Work out the finished part from the listing and answer in its coordinate system (mm). Face numbers are marked on the shaded views. A direction names the side the tool comes from. Give positions to 0.01 mm unless a question says otherwise; leave off trailing zeros. Write each loop counter-clockwise with the first axis right and the second up, starting at its lowest first coordinate (ties: lowest second). Pieces come first, ordered by that corner, then holes. Notation, with made-up numbers: (51.5, -20.5) -> (93.5, -20.5) arc R14 ccw to (93.5, -9.5) -> close; hole circle Ø5 at (63, -2). An arc over 180 degrees is marked (long way). Write item = value, one per line. Start each with the question number.
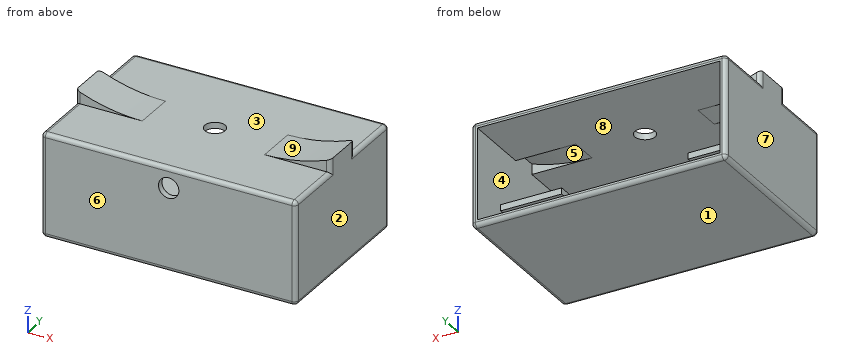
from build123d import *

# Parameters (mm, degrees)
BOSS_EXTRUDE1_DEPTH = 5
BOSS_EXTRUDE2_DEPTH = 20
SHELL1_START        = -18.5
SHELL1_OUTLINE_W    = 59.5
SHELL1_OUTLINE_H    = 22.4
SHELL1_DEPTH        = 38.5
SHELL1_START_2      = -3.5
SHELL1_2_DEPTH      = 7
SKETCH14_R          = 2.5
CUT_EXTRUDE1_DEPTH  = 1.5
SKETCH15_W          = 13.5
SKETCH15_H          = 1.5
SKETCH15_W_2        = 15
BOSS_EXTRUDE3_DEPTH = 10
FILLET21_R          = 1
CUT_EXTRUDE2_START  = -18.5
SKETCH16_R          = 2.5
CUT_EXTRUDE2_DEPTH  = 1.5


# Read off the part's stored shape, not the designer's step: Shell1
with BuildPart() as part:
    # Sketch13 → Boss-Extrude1 (new, symmetric)
    with BuildSketch(Plane(origin=(0, 0, 0), x_dir=(1, 0, 0), z_dir=(0, 1, 0))):
        with BuildLine():
            ThreePointArc((-31.25, 1.770695181), (-23.283883594, 4.184856634), (-15, 5))
            Line((-15, 5), (-31.25, 5))
            Line((-31.25, 5), (-31.25, 1.770695181))
        make_face()
        Polygon((-15, 5), (15, 5), (31.25, 5), (31.25, 30.4), (-31.25, 30.4), (-31.25, 5), align=None)
        with BuildLine():
            Line((31.25, 5), (15, 5))
            ThreePointArc((15, 5), (23.283883594, 4.184856634), (31.25, 1.770695181))
            Line((31.25, 1.770695181), (31.25, 5))
        make_face()
    extrude(amount=BOSS_EXTRUDE1_DEPTH, both=True)

    # Sketch13<12> → Boss-Extrude2 (add, symmetric)
    with BuildSketch(Plane(origin=(0, 0, 0), x_dir=(1, 0, 0), z_dir=(0, 1, 0))):
        Polygon((-15, 5), (15, 5), (31.25, 5), (31.25, 30.4), (-31.25, 30.4), (-31.25, 5), align=None)
    extrude(amount=BOSS_EXTRUDE2_DEPTH, both=True)

    # Shell1 outline → Shell1 (cut)
    with BuildSketch(Plane(origin=(0, 0, 0), x_dir=(1, 0, 0), z_dir=(0, 1, 0)).offset(SHELL1_START)):
        with Locations((0, 17.7)):
            Rectangle(SHELL1_OUTLINE_W, SHELL1_OUTLINE_H)
    extrude(amount=SHELL1_DEPTH, mode=Mode.SUBTRACT)

    # Shell1 2 outline → Shell1 2 (cut)
    with BuildSketch(Plane(origin=(0, 0, 0), x_dir=(1, 0, 0), z_dir=(0, 1, 0)).offset(SHELL1_START_2)):
        with BuildLine():
            Line((-29.75, 6.5), (-29.75, 3.954040816))
            ThreePointArc((-29.75, 3.954040816), (-22.484056523, 5.858838752), (-15, 6.5))
            Line((-15, 6.5), (-29.75, 6.5))
        make_face()
        with BuildLine():
            Line((29.75, 6.5), (15, 6.5))
            ThreePointArc((15, 6.5), (22.484056523, 5.858838752), (29.75, 3.954040816))
            Line((29.75, 3.954040816), (29.75, 6.5))
        make_face()
    extrude(amount=SHELL1_2_DEPTH, mode=Mode.SUBTRACT)

    # Sketch14 → Cut-Extrude1 (cut)
    with BuildSketch(Plane.XY.offset(-5)):
        with Locations(Location((0, 0, 0), (0, 0, 180))):
            Circle(SKETCH14_R)
    extrude(amount=-CUT_EXTRUDE1_DEPTH, mode=Mode.SUBTRACT)

    # Sketch15 → Boss-Extrude3 (add, symmetric)
    with BuildSketch(Plane(origin=(0, 0, 0), x_dir=(1, 0, 0), z_dir=(0, 1, 0))):
        with Locations((-23, 21.15)):
            Rectangle(SKETCH15_W, SKETCH15_H)
        with Locations((22.25, 21.15)):
            Rectangle(SKETCH15_W_2, SKETCH15_H)
    extrude(amount=BOSS_EXTRUDE3_DEPTH, both=True)

    # Fillet21
    fillet21_edges = [part.edges().sort_by_distance(p)[0] for p in [
        (-31.25, 0, -30.4),
        (31.25, 0, -30.4),
        (31.25, -5, -3.385347591),
        (31.25, 5, -3.385347591),
        (31.25, -12.5, -5),
        (-31.25, -20, -17.7),
        (-31.25, -12.5, -5),
        (0, -20, -5),
        (31.25, 12.5, -5),
        (31.25, 20, -17.7),
        (0, 20, -30.4),
        (-31.25, 12.5, -5),
        (-31.25, 20, -17.7),
        (0, 20, -5),
        (31.25, -20, -17.7),
        (0, -20, -30.4),
        (-31.25, 5, -3.385347591),
        (-31.25, -5, -3.385347591),
    ]]
    fillet(fillet21_edges, radius=FILLET21_R)

    # Sketch16 → Cut-Extrude2 (cut)
    with BuildSketch(Plane(origin=(0, 0, 0), x_dir=(1, 0, 0), z_dir=(0, 1, 0)).offset(CUT_EXTRUDE2_START)):
        with Locations(Location((0, 10, 0), (0, 0, 270))):
            Circle(SKETCH16_R)
    extrude(amount=-CUT_EXTRUDE2_DEPTH, mode=Mode.SUBTRACT)


solid = part.part
(1) A cutting plane is placed at C-C, the plane z = -10. Write down the section's boundary in (x, y).
(2) For the marked faces 5, 6, 7, 8 and 9, determine the directions among +Z, -Z, +X, -X, +Y, -Y from which every point of the face is accessible in a straight line to the end or side of a thin tool.
(3) Each of these flat-tipped pins is pushed along its axis until it touches: pin 1 (1.3 mm diameter, centred on x = -25.5, z = -5, fed in from +Y); pin 2 (11 mm diameter, centred on x = -22.5, y = 1.5, fed in from +Z); pin 3 (1 mm diameter, centred on x = 12.5, y = 9, fed in from +Z). Where does it stop, or does it pass through?
(4) A cutting plane is placed at A-A, the plane x = 0. Write down the section's boundary in (y, z), then the cut area to 3 significant figures.
(5) A cutting plane is placed at B-B, the plane y = -8.5. Write down the section's boundary in (x, z), then the cut area to 3 significant figures.
(6) Determine the mould class of the marked faces 1, 2, 3 and 4 for opening direction Z: pulls with the +Z half, pulls with the -Z half, needs draft (parallel to the pull), parting line crosses it, or undercut.
(7) Find the intervals of material crossed by line 1 along Z through (x, y) = (-24.5, -8.5); line 2 along Z through (x, y) = (-12.5, -7); line 3 along X through (y, z) = (14.5, -11), in increasing order.
(8) A cutting plane is placed at D-D, the plane y = 0. Write down the section's boundary in (x, z), then the cut area to 3 significant figures.
Results list:
q1.outline = (-31.25, -19) arc R1 ccw to (-30.25, -20) -> (-2.5, -20) -> (-2.5, -18.5) -> (-29.75, -18.5) -> (-29.75, 20) -> (-30.25, 20) arc R1 ccw to (-31.25, 19) -> close; (2.5, -20) -> (30.25, -20) arc R1 ccw to (31.25, -19) -> (31.25, 19) arc R1 ccw to (30.25, 20) -> (29.75, 20) -> (29.75, -18.5) -> (2.5, -18.5) -> close
q2.face_5 = none
q2.face_6 = +Z, -Z, +X, -X, -Y
q2.face_7 = +Z, -Z, -X, +Y, -Y
q2.face_8 = +Y
q2.face_9 = +Z, +Y, -Y
q3.pin_1 = 19.94
q3.pin_2 = -2.96
q3.pin_3 = -5
q4.outline = (-20, -29.4) arc R1 ccw to (-19, -30.4) -> (19, -30.4) arc R1 ccw to (20, -29.4) -> (20, -28.9) -> (-18.5, -28.9) -> (-18.5, -12.5) -> (-20, -12.5) -> close; (-20, -7.5) -> (-18.5, -7.5) -> (-18.5, -6.5) -> (-2.5, -6.5) -> (-2.5, -5) -> (-19, -5) arc R1 ccw to (-20, -6) -> close; (2.5, -6.5) -> (20, -6.5) -> (20, -6) arc R1 ccw to (19, -5) -> (2.5, -5) -> close
q4.area = 138 mm²
q5.outline = (-31.25, -29.4) arc R1 ccw to (-30.25, -30.4) -> (30.25, -30.4) arc R1 ccw to (31.25, -29.4) -> (31.25, -6) arc R1 ccw to (30.25, -5) -> (-30.25, -5) arc R1 ccw to (-31.25, -6) -> close; hole (-29.75, -28.9) -> (29.75, -28.9) -> (29.75, -21.9) -> (14.75, -21.9) -> (14.75, -20.4) -> (29.75, -20.4) -> (29.75, -6.5) -> (-29.75, -6.5) -> (-29.75, -20.4) -> (-16.25, -20.4) -> (-16.25, -21.9) -> (-29.75, -21.9) -> close
q5.area = 297 mm²
q6.face_1 = pulls with the -Z half
q6.face_2 = needs draft
q6.face_3 = pulls with the +Z half
q6.face_4 = undercut
q7.line_1 = -30.4 to -28.9, -21.9 to -20.4, -6.5 to -5
q7.line_2 = -30.4 to -28.9, -6.5 to -5
q7.line_3 = -31.25 to -29.75, 29.75 to 31.25
q8.outline = (-31.25, -29.4) arc R1 ccw to (-30.25, -30.4) -> (30.25, -30.4) arc R1 ccw to (31.25, -29.4) -> (31.25, -1.77) arc R42.5 cw to (15, -5) -> (2.5, -5) -> (2.5, -6.5) -> (15, -6.5) arc R44 ccw to (29.75, -3.95) -> (29.75, -20.4) -> (14.75, -20.4) -> (14.75, -21.9) -> (29.75, -21.9) -> (29.75, -28.9) -> (-29.75, -28.9) -> (-29.75, -21.9) -> (-16.25, -21.9) -> (-16.25, -20.4) -> (-29.75, -20.4) -> (-29.75, -3.95) arc R44 ccw to (-15, -6.5) -> (-2.5, -6.5) -> (-2.5, -5) -> (-15, -5) arc R42.5 cw to (-31.25, -1.77) -> close
q8.area = 299 mm²
